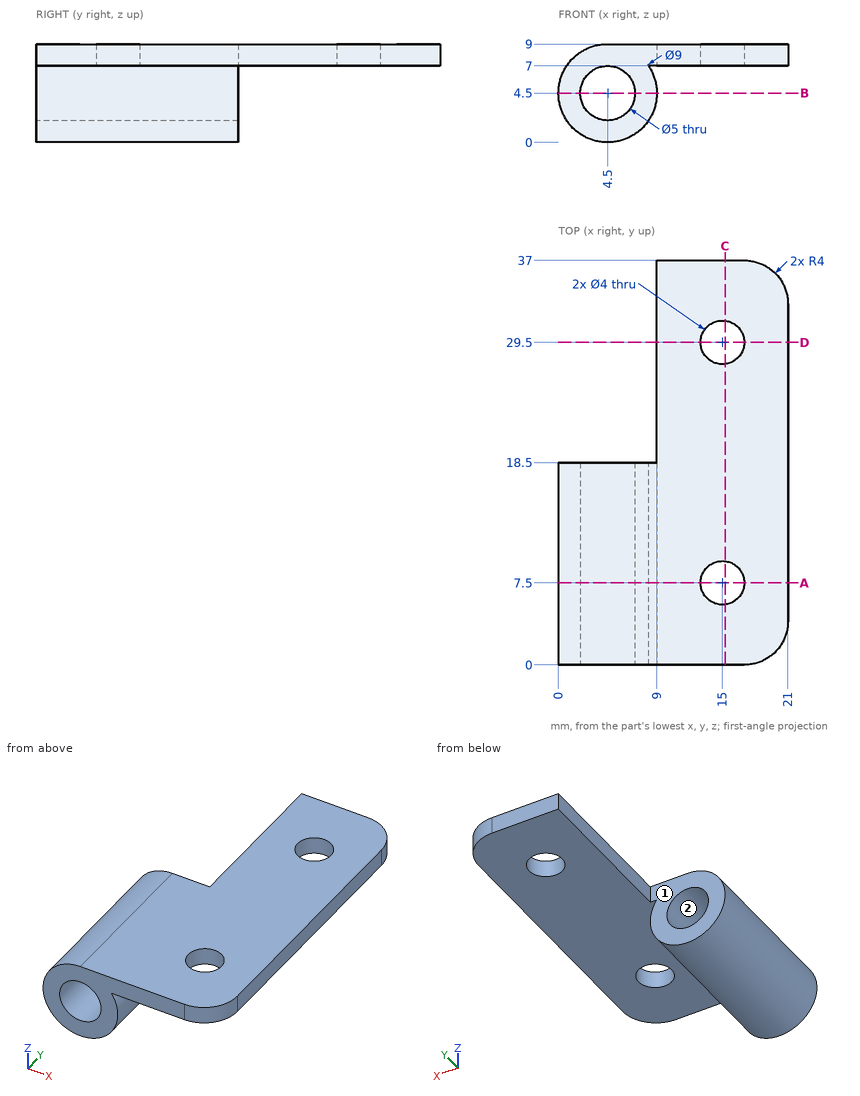
Answer from the drawing. Dimensions are ordinates in mm from the lowest x, y and z of the part. Give positions to 0.01 mm unless a question says otherwise; leave off trailing zeros. Loops run counter-clockwise (first coordinate to the right, second up) from the corner with the lowest first, then second, coordinate; pieces in that order, holes last. Notation, with made-up numbers: (-20.5, -20) -> (2.5, -20) arc R17 cw to (2.5, 12) -> close; hole circle Ø4 at (88, 7). An arc over 180 degrees is marked (long way). Answer as CSV lines item,"result".
Item 1: Consider line 1 (Y direction, x = 15, z = 8.1); line 2 (X direction, y = 6.5, z = 4.5); line 3 (Y direction, x = 8.5, z = 4.5). Determine where each line is inside the solid, lowest interval first. Write a range as [from, to].
Returned:
line 1,"y = [0, 5.5], [9.5, 27.5], [31.5, 37]"
line 2,"x = [0, 2], [7, 9]"
line 3,"y = [0, 18.5]"
Item 2: Determine the mould class of the marked faces 1 and 2 for opening direction X: +X half, -X half, draft (parallel to the pull), parting line (faces both ways), or undercut.
Returned:
face 1,"draft"
face 2,"undercut"
Item 3: Find section B-B on z = 4.5. Give the vertices of the cut face in (x, y), plus the area to 3 significant figures.
Returned:
outline,"(0, 0) -> (2, 0) -> (2, 18.5) -> (0, 18.5) -> close; (7, 0) -> (9, 0) -> (9, 18.5) -> (7, 18.5) -> close"
area,"74.0 mm²"
Item 4: Find section C-C on x = 15.25. Give the vertices of the cut face in (y, z).
Returned:
outline,"(0, 7) -> (5.52, 7) -> (5.52, 9) -> (0, 9) -> close; (9.48, 7) -> (27.52, 7) -> (27.52, 9) -> (9.48, 9) -> close; (31.48, 7) -> (37, 7) -> (37, 9) -> (31.48, 9) -> close"
Item 5: Each of these flat-tipped pins is pushed along its axis until it touches: pin 1 (3 mm diameter, centred on x = 4.5, z = 4.5, fed in from -Y); pin 2 (5 mm diameter, centred on x = 15, y = 7.5, fed in from -Z); pin 3 (1 mm diameter, centred on y = 25.5, z = 8, fed in from -X); pin 4 (5 mm diameter, centred on y = 19, z = 3.5, fed in from +X). Where does it stop, or does it pass through?
Returned:
pin 1,"passes through"
pin 2,"stops at z = 7"
pin 3,"stops at x = 9"
pin 4,"stops at x = 9"
Item 6: Find section A-A on y = 7.5. Give the vertices of the cut face in (x, z), plus the area to 3 significant figures.
Returned:
outline,"(4.5, 9) arc R4.5 ccw (long way) to (8.24, 7) -> (13, 7) -> (13, 9) -> close; (17, 7) -> (21, 7) -> (21, 9) -> (17, 9) -> close; hole circle Ø5 at (4.5, 4.5)"
area,"63.7 mm²"
Item 7: Find section D-D on y = 29.5. Give the vertices of the cut face in (x, z), plus the area to 3 significant figures.
Returned:
outline,"(9, 7) -> (13, 7) -> (13, 9) -> (9, 9) -> close; (17, 7) -> (21, 7) -> (21, 9) -> (17, 9) -> close"
area,"16.0 mm²"
